```python
from build123d import *

# Parameters (mm, degrees)
F0_W     = 57.15
F0_H     = 88.9
F1_DEPTH = 3.175
F2_W     = 3.175
F2_H     = 88.9
F3_DEPTH = 50.8
F4_W     = 3.175
F4_H     = 88.9
F5_DEPTH = 50.8
F6_W     = 3.175
F6_H     = 88.9
F7_DEPTH = 50.8


with BuildPart() as f1:
    # F0 (on Front) → F1 (new body)
    with BuildSketch(Plane.XZ):
        with Locations((-4.401278, 4.662237)):
            Rectangle(F0_W, F0_H)
    extrude(amount=F1_DEPTH)

    # F2 (on face) → F3 (join)
    with BuildSketch(Plane.XZ.offset(3.175)):
        with Locations((22.586222, 4.662237)):
            Rectangle(F2_W, F2_H)
    extrude(amount=F3_DEPTH)

    # F4 (on face) → F5 (join)
    with BuildSketch(Plane.XZ.offset(3.175)):
        with Locations((-31.388778, 4.662237)):
            Rectangle(F4_W, F4_H)
    extrude(amount=F5_DEPTH)

    # F6 (on face) → F7 (join)
    with BuildSketch(Plane.YZ.offset(-29.801278)):
        with Locations((-52.3875, 4.662237)):
            Rectangle(F6_W, F6_H)
    extrude(amount=F7_DEPTH)


solid = f1.part
```
Design review of the part built by this model. Coordinates are the model's own, in mm. A direction names the side the tool comes from. Give positions to 0.01 mm unless a question says otherwise; leave off trailing zeros. Order: outer loops, then holes, each group sorted by start corner. A loop starts at its lowest first (then second) coordinate and runs counter-clockwise, first axis right, second up. Notation, with made-up numbers: M 74,35 L 99,35 A21 ccw 99,47 Z; hole C 14.5,-6 d2. An arc over 180 degrees is marked long. One line per question, with ' | ' between items. Start each with the question number.
Q1. Machinability: for faces 4 (the face through (-5, -3.175, 5)), 5 (the face through (-32.976, -27, 4)), which of the approach directions +Z, -Z, +X, -X, +Y, -Y give a long, thin tool a straight path to every point of the face, cutting with its end or side? Answer none if there is none.
Q2. For L1, parallel to X at y = -49.5, z = 0; L2, parallel to Y at x = -28.5, z = 39.5 (3 decimals), list the stretches that pass through material, from the lowest coordinate up. Write a range as [from, to].
Q3. We need section C-C (z = 27.5). Write out the cut boundary in (x, y) (3 decimals).
Q4. We need section A-A (x = -28.5). Write out the cut boundary in (y, z) (3 decimals), plus the area to 3 significant figures.
Q5. We need section B-B (y = -22.5). Write out the cut boundary in (x, z), plus the area to 3 significant figures.
Q6. The part is to be moulded in two halves that separate along Y. For faces 1 (the face through (-30, -27, 49.112)), 2 (the face through (-5, 0, 5)), 3 (the face through (-5, -50.8, 4)), say which applies: +Y half, -Y half, draft (parallel to the pull), parting line (faces both ways), or undercut.
Returned:
1) face 4: +Z, -Z | face 5: +Z, -Z, -X, +Y, -Y
2) L1: [-32.98, -29.8], [21, 24.17] | L2: [-53.975, -50.8], [-3.175, 0]
3) outline: M -32.976,-53.975 L 24.174,-53.975 L 24.174,0 L -32.976,0 Z; hole M -29.801,-50.8 L 20.999,-50.8 L 20.999,-3.175 L -29.801,-3.175 Z
4) outline: M -53.975,-39.788 L -50.8,-39.788 L -50.8,49.112 L -53.975,49.112 Z; M -3.175,-39.788 L 0,-39.788 L 0,49.112 L -3.175,49.112 Z | area: 565 mm2
5) outline: M -32.98,-39.79 L -29.8,-39.79 L -29.8,49.11 L -32.98,49.11 Z; M 21,-39.79 L 24.17,-39.79 L 24.17,49.11 L 21,49.11 Z | area: 565 mm2
6) face 1: draft | face 2: +Y half | face 3: undercut
